```python
from build123d import *
from build123d.topology import SkipClean

# Parameters (mm, degrees)
SKETCH_1_W          = 47
SKETCH_1_H          = 93.5
SKETCH_1_R          = 1.5
SKETCH_1_W_2        = 18
SKETCH_1_H_2        = 12
EXTRUDE_1_DEPTH     = 4
EXTRUDE_START       = 1
SKETCH_3_W          = 8
SKETCH_3_H          = 8
SKETCH_3_R          = 1.5
EXTRUDE_2_DEPTH     = 1
SKETCH_4_R          = 1.5
SKETCH_4_W          = 47
SKETCH_4_H          = 5
CUT_EXTRUDE_2_DEPTH = 4


with BuildPart() as part:
    # 草图1 → 凸台-拉伸1 (new body)
    with BuildSketch(Plane(origin=(0, 0, 0), x_dir=(1, 0, 0), z_dir=(0, 1, 0))):
        with Locations((0, -26.75)):
            Rectangle(SKETCH_1_W, SKETCH_1_H)
        with Locations(Location((-19.5, -14, 0), (0, 0, 270))):
            Circle(SKETCH_1_R, mode=Mode.SUBTRACT)
        with Locations((6, -12)):
            Rectangle(SKETCH_1_W_2, SKETCH_1_H_2, mode=Mode.SUBTRACT)
        with Locations(Location((-19.5, 14, 0), (0, 0, 270))):
            Circle(SKETCH_1_R, mode=Mode.SUBTRACT)
        with Locations(Location((19.5, -14, 0), (0, 0, 270))):
            Circle(SKETCH_1_R, mode=Mode.SUBTRACT)
        with Locations(Location((19.5, 14, 0), (0, 0, 270))):
            Circle(SKETCH_1_R, mode=Mode.SUBTRACT)
    extrude(amount=EXTRUDE_1_DEPTH)

    # 草图3 → 凸台-拉伸2 (add)
    # profile 1 of 4: a face of its own
    with SkipClean():  # the faces are left unmerged after this step: merging them gives an invalid solid
        with BuildSketch(Plane.XZ.offset(EXTRUDE_START)):
            with Locations((19.5, -14)):
                Rectangle(SKETCH_3_W, SKETCH_3_H)
            with Locations(Location((19.5, -14, 0), (0, 0, 270))):
                Circle(SKETCH_3_R, mode=Mode.SUBTRACT)
        # profile 2 of 4: a face of its own
        with BuildSketch(Plane.XZ.offset(EXTRUDE_START)):
            with Locations((19.5, 14)):
                Rectangle(SKETCH_3_W, SKETCH_3_H)
            with Locations(Location((19.5, 14, 0), (0, 0, 270))):
                Circle(SKETCH_3_R, mode=Mode.SUBTRACT)
        # profile 3 of 4: a face of its own
        with BuildSketch(Plane.XZ.offset(EXTRUDE_START)):
            with Locations((-19.5, -14)):
                Rectangle(SKETCH_3_W, SKETCH_3_H)
            with Locations(Location((-19.5, -14, 0), (0, 0, 270))):
                Circle(SKETCH_3_R, mode=Mode.SUBTRACT)
        # profile 4 of 4: a face of its own
        with BuildSketch(Plane.XZ.offset(EXTRUDE_START)):
            with Locations((-19.5, 14)):
                Rectangle(SKETCH_3_W, SKETCH_3_H)
            with Locations(Location((-19.5, 14, 0), (0, 0, 270))):
                Circle(SKETCH_3_R, mode=Mode.SUBTRACT)
        extrude(amount=-EXTRUDE_2_DEPTH)

    # 草图4 → 切除-拉伸2 (cut)
    with SkipClean():  # the faces are left unmerged after this step: merging them gives an invalid solid
        with BuildSketch(Plane(origin=(0, 4, 0), x_dir=(1, 0, 0), z_dir=(0, 1, 0))):
            with Locations(Location((9, -28.5, 0), (0, 0, 270))):
                Circle(SKETCH_4_R)
            with Locations(Location((9, -48.5, 0), (0, 0, 270))):
                Circle(SKETCH_4_R)
            with Locations(Location((-9, -48.5, 0), (0, 0, 90))):
                Circle(SKETCH_4_R)
            with Locations(Location((-9, -28.5, 0), (0, 0, 90))):
                Circle(SKETCH_4_R)
            with Locations(Location((-9, -36.5, 0), (0, 0, 90))):
                Circle(SKETCH_4_R)
            with Locations(Location((9, -36.5, 0), (0, 0, 270))):
                Circle(SKETCH_4_R)
            with Locations(Location((9, -56.5, 0), (0, 0, 270))):
                Circle(SKETCH_4_R)
            with Locations(Location((-9, -56.5, 0), (0, 0, 90))):
                Circle(SKETCH_4_R)
            with Locations((0, -71)):
                Rectangle(SKETCH_4_W, SKETCH_4_H)
        extrude(amount=-CUT_EXTRUDE_2_DEPTH, mode=Mode.SUBTRACT)


solid = part.part
```
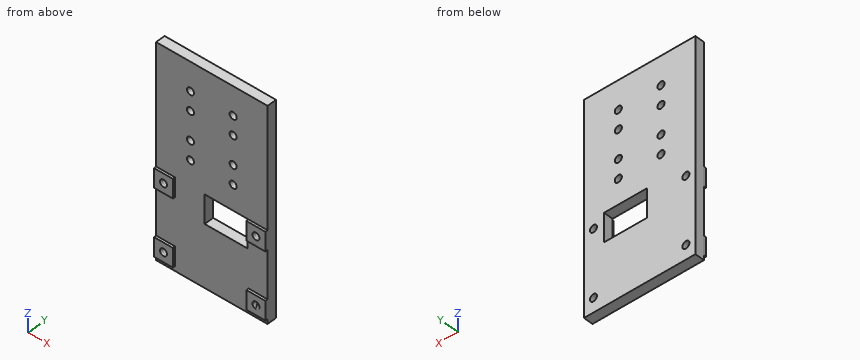
The listing builds one solid part. Answer for the finished solid, in the listing's coordinates (mm). Give positions to 0.01 mm unless a question says otherwise; leave off trailing zeros. Write each loop counter-clockwise with the first axis right and the second up, starting at its lowest first coordinate (ties: lowest second). Pieces come first, ordered by that corner, then holes. Notation, with made-up numbers: M -28.5,82 L -13.5,82 A17 cw -13.5,110 Z; hole C -39,-26.75 d3. An arc over 180 degrees is marked long. Write each question's results on one line, items separated by ' | '.
Q1. Section A-A, the plane x = 9 is taken. Write down the section's boundary in (y, z), then the cut area to 3 significant figures.
Output values:
outline: M 0,-20 L 4,-20 L 4,6 L 0,6 Z; M 0,18 L 4,18 L 4,27 L 0,27 Z; M 0,30 L 4,30 L 4,35 L 0,35 Z; M 0,38 L 4,38 L 4,47 L 0,47 Z; M 0,50 L 4,50 L 4,55 L 0,55 Z; M 0,58 L 4,58 L 4,68.5 L 0,68.5 Z | area: 258 mm2
Q2. Section C-C, the plane z = 14 is taken. Write down the section's boundary in (x, y).
Output values:
outline: M -23.5,-1 L -21,-1 L -21,4 L -23.5,4 Z; M -18,-1 L -15.5,-1 L -15.5,0 L -3,0 L -3,4 L -18,4 Z; M 15,0 L 15.5,0 L 15.5,-1 L 18,-1 L 18,4 L 15,4 Z; M 21,-1 L 23.5,-1 L 23.5,4 L 21,4 Z
Q3. Section D-D, the plane z = 28.5 is taken. Write down the section's boundary in (x, y).
Output values:
outline: M -23.5,0 L -10.5,0 L -10.5,4 L -23.5,4 Z; M -7.5,0 L 7.5,0 L 7.5,4 L -7.5,4 Z; M 10.5,0 L 23.5,0 L 23.5,4 L 10.5,4 Z
Q4. Flat-ended cylindrical pins translate along their axes: P1, Ø5, axis at x = -11.5, z = 43, coming from the -Y side; P2, Ø2.5, axis at x = 9, z = 36.5, coming from the +Y side; P3, Ø0.5, axis at x = 19, y = -0.5, coming from the -Z side. Find the tip coordinate at first contact, or state that the pin passes through.
Output values:
P1: y = 0 | P2: through | P3: z = -18
Q5. Consider L1, parallel to X at y = 1.3, z = 14; L2, parallel to X at y = 2.7, z = -14; L3, parallel to X at y = 1.95, z = 56.5. Determine where each line is inside the solid, lowest interval first. Write a range as from..to.
Output values:
L1: -23.5..-21, -18..-3, 15..18, 21..23.5 | L2: -23.5..-21, -18..18, 21..23.5 | L3: -23.5..-10.5, -7.5..7.5, 10.5..23.5
Q6. Section B-B, the plane x = -19.5 is taken. Write down the section's boundary in (y, z).
Output values:
outline: M -1,-18 L 0,-18 L 0,-20 L 4,-20 L 4,-15.5 L -1,-15.5 Z; M -1,-12.5 L 4,-12.5 L 4,12.5 L -1,12.5 L -1,10 L 0,10 L 0,-10 L -1,-10 Z; M -1,15.5 L 4,15.5 L 4,68.5 L 0,68.5 L 0,18 L -1,18 Z
